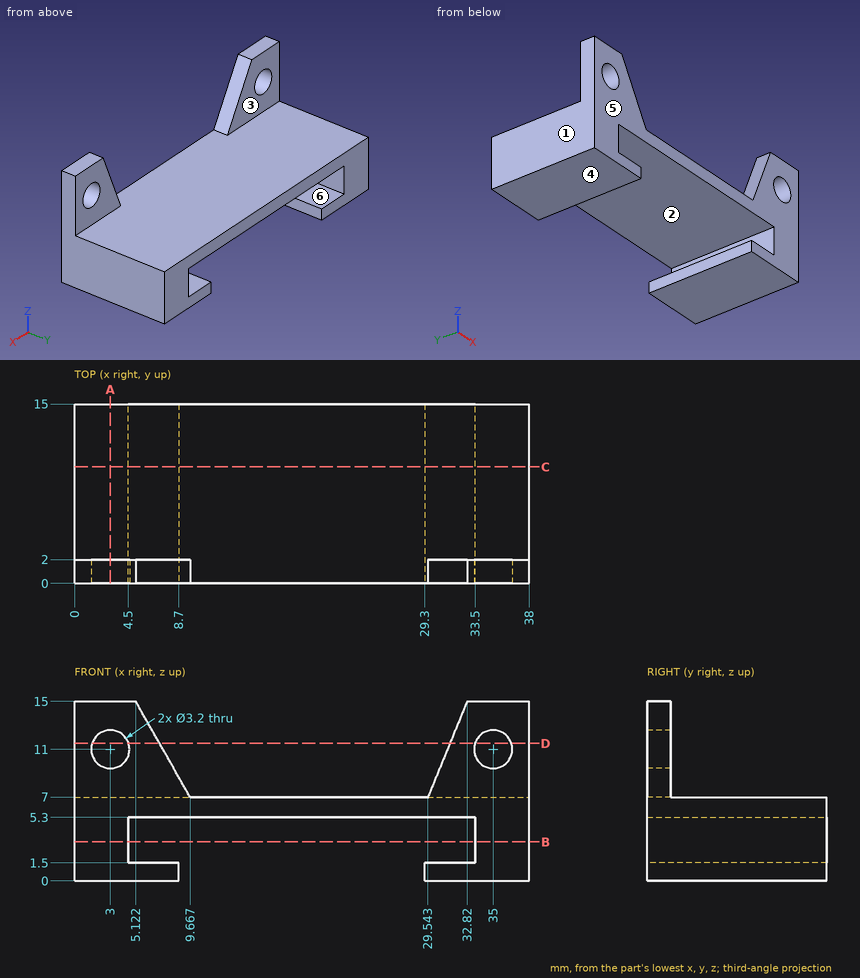
Study the drawing (mm; zero at the part's minimum x, y, z) and answer. A direction names the side the tool comes from. Give positions to 0.01 mm unless a question says otherwise; leave off trailing zeros. Write each loop counter-clockwise with the first axis right and the second up, starting at its lowest first coordinate (ties: lowest second). Pieces come first, ordered by that corner, then holes.
(1) The part is cut by section B-B on z = 3.25. Write down the section's boundary in (x, y), plus the area to 3 significant figures.
Final values:
outline: (0, 0) - (4.5, 0) - (4.5, 15) - (0, 15) - close; (33.5, 0) - (38, 0) - (38, 15) - (33.5, 15) - close
area: 135 mm2
(2) Flat-ended cylindrical pins translate along their axes: pin 1 Ø1.9 at (x, z) = (35, 11) entering from +Y; pin 2 Ø4.5 at (x, y) = (6, 5) entering from +Z; pin 3 Ø5 at (x, z) = (32, 12) entering from +Y; pin 4 Ø7.5 at (x, y) = (19, 6.5) entering from -Z. Find the tip coordinate at first contact, or state that the pin passes through.
Final values:
pin 1: passes through
pin 2: stops at z = 7
pin 3: stops at y = 2
pin 4: stops at z = 5.3
(3) Which of the six approach directions +Z, -Z, +X, -X, +Y, -Y give full straight-line access (tool end or side, diameter ignored) to the marked faces 1, 2 and 3?
Final values:
face 1: +Z, -Z, -X, +Y, -Y
face 2: +Y, -Y
face 3: +Z, +X, -X, +Y
(4) Straight lines are drawn through the part: line 1 (X direction, y = 6.5, z = 3); line 2 (Z direction, x = 3, y = 0.9); line 3 (Z direction, x = 6.5, y = 13.5). For each, find the intervals that lie inside material, in ascending order.
Final values:
line 1: x = 0 to 4.5, 33.5 to 38
line 2: z = 0 to 9.4, 12.6 to 15
line 3: z = 0 to 1.5, 5.3 to 7
(5) The mould has two halves that part along Z. Classify the marked faces 4, 5 and 6: pulls with the +Z half, pulls with the -Z half, needs draft (parallel to the pull), parting line crosses it, or undercut.
Final values:
face 4: pulls with the -Z half
face 5: needs draft
face 6: undercut
(6) The part is cut by section D-D on z = 11.5. Write down the section's boundary in (x, y), plus the area to 3 significant figures.
Final values:
outline: (0, 0) - (1.48, 0) - (1.48, 2) - (0, 2) - close; (4.52, 0) - (7.11, 0) - (7.11, 2) - (4.52, 2) - close; (31.39, 0) - (33.48, 0) - (33.48, 2) - (31.39, 2) - close; (36.52, 0) - (38, 0) - (38, 2) - (36.52, 2) - close
area: 15.3 mm2
(7) The part is cut by section C-C on y = 9.75. Write down the section's boundary in (x, z), plus the area to 3 significant figures.
Final values:
outline: (0, 0) - (8.7, 0) - (8.7, 1.5) - (4.5, 1.5) - (4.5, 5.3) - (33.5, 5.3) - (33.5, 1.5) - (29.3, 1.5) - (29.3, 0) - (38, 0) - (38, 7) - (0, 7) - close
area: 125 mm2
(8) The part is cut by section A-A on x = 3. Write down the section's boundary in (y, z).
Final values:
outline: (0, 0) - (15, 0) - (15, 7) - (2, 7) - (2, 9.4) - (0, 9.4) - close; (0, 12.6) - (2, 12.6) - (2, 15) - (0, 15) - close
